from build123d import *

# Parameters (mm, degrees)
BOSS_EXTRUDE1_DEPTH     = 79.29
FILLET1_R               = 1
FILLET2_R               = 2
SKETCH2_R               = 1.6
CUT_EXTRUDE1_DEPTH      = 308.8152925
CUT_EXTRUDE4_DEPTH      = 308.8152925
CUT_EXTRUDE4_DEPTH_BACK = 308.8152925


with BuildPart() as part:
    # Sketch1 → Boss-Extrude1 (new body)
    with BuildSketch(Plane.XY):
        Polygon((293.529130065, -14.271367807), (293.529130065, -64.271367807), (281.529130065, -64.271367807), (281.529130065, -62.271367807), (291.529130065, -62.271367807), (291.529130065, -14.271367807), align=None)
    extrude(amount=BOSS_EXTRUDE1_DEPTH)

    # Fillet1
    fillet1_edges = [part.edges().sort_by_distance(p)[0] for p in [
        (281.529130065, -62.271367807, 39.645),
        (291.529130065, -14.271367807, 39.645),
    ]]
    fillet(fillet1_edges, radius=FILLET1_R)

    # Fillet2
    fillet2_edges = [part.edges().sort_by_distance(p)[0] for p in [
        (291.529130065, -62.271367807, 39.645),
    ]]
    fillet(fillet2_edges, radius=FILLET2_R)

    # Sketch2 → Cut-Extrude1 (cut, through all)
    with BuildSketch(Plane(origin=(0, -62.271367807, 0), x_dir=(1, 0, 0), z_dir=(0, 1, 0))):
        with Locations(Location((286.029130065, -20, 0), (0, 0, 270))):
            Circle(SKETCH2_R)
        with Locations(Location((286.029130065, -59.29, 0), (0, 0, 270))):
            Circle(SKETCH2_R)
    extrude(amount=-CUT_EXTRUDE1_DEPTH, mode=Mode.SUBTRACT)

    # Sketch3 → Cut-Extrude4 (cut, two sides: drawn at the far end of the back side and taken through both)
    with BuildSketch(Plane(origin=(0, -62.271367807, 0), x_dir=(1, 0, 0), z_dir=(0, 1, 0)).offset(-CUT_EXTRUDE4_DEPTH_BACK)):
        Polygon((293.529130065, 0), (281.33161049, -12.197519575), (281.33161049, 1.118185929), (293.529130065, 1.118185929), align=None)
    extrude(amount=CUT_EXTRUDE4_DEPTH + CUT_EXTRUDE4_DEPTH_BACK, mode=Mode.SUBTRACT)


solid = part.part
Verification items for the finished model (mm, model axes). A direction names the side the tool comes from. Coordinates: 2 decimals unless noted, no trailing zeros. Write each loop counter-clockwise with the first axis right and the second up, starting at its lowest first coordinate (ties: lowest second). Pieces come first, ordered by that corner, then holes. Notation, with made-up numbers: M -11.5,50.5 L 41.5,50.5 A18 ccw 41.5,75.5 Z; hole C 1.25,25.25 d5. An arc over 180 degrees is marked long. One line per question, with ' | ' between items.
1) Release check for a two-part mould opening along X. For faces 1 (the face through (293.529, -39, 39)), 2 (the face through (291.529, -38, 40)), 3 (the face through (284.467, -63.257, 19.653)) record: +X half, -X half, draft (parallel to the pull), parting line (faces both ways), or undercut.
Solutions:
face 1: +X half | face 2: -X half | face 3: undercut
2) Depth check by flat-ended pin: pin 1 Ø2 at (x, z) = (287.5, 27) entering from +Y. Enter the tip coordinate at first touch or a pass-through.
Solutions:
pin 1: y = -62.27
3) Access from +Z, -Z, +X, -X, +Y, -Y to the whole of each face (thin tool, end or side, straight path). Record for faces 4 (the face through (292, -43, 79.29)), 5 (the face through (286, -62.271, 41)).
Solutions:
face 4: +Z, +X, -X, +Y, -Y | face 5: +Z, -Z, -X, +Y
4) Sectioned sample at A-A on z = 20. Record the cut outline in (x, y), then the cut area to 3 significant figures.
Solutions:
outline: M 281.53,-64.27 L 284.43,-64.27 L 284.43,-62.27 L 282.53,-62.27 A1 ccw 281.53,-63.27 Z; M 287.63,-64.27 L 293.53,-64.27 L 293.53,-14.27 L 292.53,-14.27 A1 ccw 291.53,-15.27 L 291.53,-60.27 A2 cw 289.53,-62.27 L 287.63,-62.27 Z | area: 114 mm^2
5) Sectioned sample at B-B on z = 42. Record the cut outline in (x, y).
Solutions:
outline: M 281.53,-64.27 L 293.53,-64.27 L 293.53,-14.27 L 292.53,-14.27 A1 ccw 291.53,-15.27 L 291.53,-60.27 A2 cw 289.53,-62.27 L 282.53,-62.27 A1 ccw 281.53,-63.27 Z
6) Material ranges on L1, parallel to X at y = -63.7, z = 20; L2, parallel to X at y = -62.8, z = 20; L3, parallel to X at y = -17.5, z = 48.5, recorded low to high.
Solutions:
L1: 281.53 to 284.43, 287.63 to 293.53 | L2: 281.65 to 284.43, 287.63 to 293.53 | L3: 291.53 to 293.53
7) Sectioned sample at D-D on x = 290.5. Record the cut outline in (y, z), then the cut area to 3 significant figures.
Solutions:
outline: M -64.27,3.03 L -62.02,3.03 L -62.02,79.29 L -64.27,79.29 Z | area: 172 mm^2
8) Sectioned sample at C-C on y = -24. Record the cut outline in (x, z), then the cut area to 3 significant figures.
Solutions:
outline: M 291.53,2 L 293.53,0 L 293.53,79.29 L 291.53,79.29 Z | area: 157 mm^2
